Autodesk Inventor part; units mm, degrees
ref_plane "YZ Plane" through (0, 0, 0) normal (1, 0, 0) x (0, 1, 0)
ref_plane "XZ Plane" through (0, 0, 0) normal (0, 1, 0) x (-1, 0, 0)
ref_plane "XY Plane" through (0, 0, 0) normal (0, 0, 1) x (1, 0, 0)
sketch "Sketch1" plane through (0, 0, 0) normal (0, 1, 0) x (-1, 0, 0)
  line L0 (7.0328, 27.6191) -> (-5.6672, 27.6191)
  line L1 (-5.6672, 27.6191) -> (-5.6672, -129.8609)
  line L2 (-5.6672, -129.8609) -> (7.0328, -129.8609)
  line L3 (7.0328, -129.8609) -> (7.0328, 27.6191)
  point P0 (0, 0)
  dimension "d0" = 12.7
  dimension "d1" = 157.48
extrude "Extrusion1" add sketch "Sketch1" along normal blind 69.85
sketch "Sketch2" plane through (-7.0328, 0, 27.6191) normal (0, 0, 1) x (1, 0, 0)
  line L0 (12.7, 0) -> (12.7, 69.85)
  line L1 (12.7, 0) -> (0, 0)
  line L2 (0, 69.85) -> (12.7, 69.85)
  point P0 (7.0328, 0)
  point P1 (6.35, 57.15)
  point P2 (6.35, 12.7)
  dimension "d4" = 0
  dimension "d5" = 6.35
  dimension "d6" = 12.7
  dimension "d7" = 12.7
hole "Hole1" at (-0.6828, 57.15, 27.6191) at (-0.6828, 12.7, 27.6191) direction (0, 0, -1) diameter 4.318 end through all
sketch "Sketch3" plane through (0, 69.85, 0) normal (0, 1, 0) x (1, 0, 0)
  line L0 (-7.0328, 129.8609) -> (-7.0328, -27.6191)
  line L1 (-7.0328, -27.6191) -> (5.6672, -27.6191)
  line L2 (5.6672, 129.8609) -> (-7.0328, 129.8609)
  point P0 (0, 0)
  point P1 (-0.6828, 23.1809)
  point P2 (-0.6828, 23.0627)
  point P3 (-0.6828, 79.0609)
  dimension "d15" = 0
  dimension "d16" = 6.35
  dimension "d17" = 50.8
  dimension "d18" = 50.8
  dimension "d26" = 55.88
hole "Hole2" at (-0.6828, 69.85, -23.1809) at (-0.6828, 69.85, -23.0627) at (-0.6828, 69.85, -79.0609) direction (0, -1, 0) diameter 4.318 end through all
properties part number "BatterySide"
The model under review builds one solid part; all positions refer to its coordinate system, in mm. A direction names the side the tool comes from. Round coordinates to 2 decimals unless told otherwise and drop trailing zeros. Loops run counter-clockwise (first coordinate to the right, second up) from the corner with the lowest first, then second, coordinate; pieces in that order, holes last. Notation, with made-up numbers: (16.25, 27.25) - (64.25, 27.25) arc R30 ccw to (64.25, 56.25) - close; hole circle Ø8 at (82, -23.5). An arc over 180 degrees is marked (long way). Use CSV: the item, a comma, the result in double quotes.
(1) Machinability: for faces 4 (the cylindrical face through (-0.634, 6.261, -20.904)), 5 (the flat face through (-7.033, 34, -52)), which of the approach directions +Z, -Z, +X, -X, +Y, -Y give a long, thin tool a straight path to every point of the face, cutting with its end or side? Answer none if there is none.
Working result:
face 4,"+Y, -Y"
face 5,"+Z, -Z, -X, +Y, -Y"
(2) Clearance check with a flat-ended pin moving along its axis: P1, Ø5.5, axis at x = -0.68, y = 57.15, coming from the +Z side. State where the tip first meets the part, or that it passes through.
Working result:
P1,"stops at z = 27.62"
(3) For line 1 (Y direction, x = -1, z = -101.5); line 2 (Y direction, x = 0.25, z = -56); line 3 (Z direction, x = 0.5, y = 54.5), list the stretches that pass through material, from the lowest coordinate up.
Working result:
line 1,"y = 0 to 10.56, 14.84 to 55.01, 59.29 to 69.85"
line 2,"y = 0 to 10.75, 14.65 to 55.2, 59.1 to 69.85"
line 3,"z = -129.86 to -80.87, -77.25 to -24.99, -21.26 to 27.62"
(4) The part is to be moulded in two halves that separate along Z. For faces 1 (the cylindrical face through (-2.142, 14.291, -104.816)), 2 (the cylindrical face through (-0.73, 34.61, -25.34)), 3 (the flat face through (-1, 34, 27.619)), say which applies: pulls with the +Z half, pulls with the -Z half, needs draft (parallel to the pull), parting line crosses it, or undercut.
Working result:
face 1,"needs draft"
face 2,"undercut"
face 3,"pulls with the +Z half"
(5) Take a section at A-A, the plane z = 6. Give the boundary of the cut face in (x, y).
Working result:
outline,"(-7.03, 0) - (5.67, 0) - (5.67, 69.85) - (-7.03, 69.85) - close; hole circle Ø4.32 at (-0.68, 12.7); hole circle Ø4.32 at (-0.68, 57.15)"
